Could you check a few things on this model? Use its own coordinates, in mm. A direction names the side the tool comes from. Round coordinates to 2 decimals unless told otherwise and drop trailing zeros. Loops run counter-clockwise (first coordinate to the right, second up) from the corner with the lowest first, then second, coordinate; pieces in that order, holes last. Notation, with made-up numbers: (22, 38) -> (74, 38) arc R21 cw to (74, 55) -> close; hole circle Ø5 at (21.5, -34). An arc over 180 degrees is marked (long way). One line per item, written item: value.
from build123d import *

# Parameters (mm, degrees)
BOSS_EXTRUDE1_DEPTH      = 17
SKETCH4_W                = 2.55
SKETCH4_H                = 15.3
SKETCH4_H_2              = 13.3
BOSS_EXTRUDE4_DEPTH      = 5
CHAMFER1_SIZE            = 0.6
SKETCH2_W                = 27.1
SKETCH2_H                = 15.3
BOSS_EXTRUDE2_DEPTH      = 2
SKETCH3_R                = 2.4
BOSS_EXTRUDE3_DEPTH      = 6
SKETCH5_R                = 0.75
CUT_EXTRUDE1_DEPTH       = 6
CUT_EXTRUDE2_REACH       = 41.661
SKETCH7_W                = 10
SKETCH7_H                = 2
BOSS_EXTRUDE5_DEPTH      = 45
BOSS_EXTRUDE5_DEPTH_BACK = 45
BOSS_EXTRUDE6_START      = -2
BOSS_EXTRUDE6_DEPTH      = 2
CHAMFER2_SIZE            = 0.6
CHAMFER4_SIZE            = 1
CHAMFER5_SIZE            = 0.8
BOSS_EXTRUDE7_START      = -3
BOSS_EXTRUDE7_DEPTH      = 3.6
LPATTERN1_COUNT          = 7
LPATTERN1_PITCH          = 14.6
FILLET1_R                = 5


with BuildPart() as part:
    # Sketch1 → Boss-Extrude1 (new body)
    with BuildSketch(Plane(origin=(0, 0, 0), x_dir=(1, 0, 0), z_dir=(0, 1, 0))):
        Polygon((-6.3, 5.3), (-6.3, -7), (-8.3, -7), (-8.3, 8.3), (18.8, 8.3), (18.8, -7), (16.8, -7), (16.8, 5.3), align=None)
    extrude(amount=-BOSS_EXTRUDE1_DEPTH)

    # Sketch4 → Boss-Extrude4 (add)
    with BuildSketch(Plane(origin=(0, 0, 0), x_dir=(1, 0, 0), z_dir=(0, 1, 0))):
        with Locations((-9.575, 0.65)):
            Rectangle(SKETCH4_W, SKETCH4_H)
        with Locations((20.075, -0.35)):
            Rectangle(SKETCH4_W, SKETCH4_H_2)
    extrude(amount=-BOSS_EXTRUDE4_DEPTH)

    # Chamfer1
    chamfer1_edges = [part.edges().sort_by_distance(p)[0] for p in [
        (16.8, 0, 0.85),
        (5.25, 0, -5.3),
        (-6.3, 0, 0.85),
    ]]
    chamfer(chamfer1_edges, length=CHAMFER1_SIZE)

    # Sketch2 → Boss-Extrude2 (add)
    with BuildSketch(Plane.XZ.offset(17)):
        with Locations((5.25, -0.65)):
            Rectangle(SKETCH2_W, SKETCH2_H)
    extrude(amount=BOSS_EXTRUDE2_DEPTH)

    # Sketch3 → Boss-Extrude3 (add)
    with BuildSketch(Plane.XZ.offset(19)):
        with Locations(Location((0, 1, 0), (0, 0, 270))):
            Circle(SKETCH3_R)
    extrude(amount=BOSS_EXTRUDE3_DEPTH)

    # Sketch5 → Cut-Extrude1 (cut)
    with BuildSketch(Plane(origin=(0, 0, 0), x_dir=(1, 0, 0), z_dir=(0, 1, 0))):
        with Locations(Location((-8.55, -1, 0), (0, 0, 270))):
            Circle(SKETCH5_R)
        with Locations(Location((19.05, -1, 0), (0, 0, 270))):
            Circle(SKETCH5_R)
    extrude(amount=-CUT_EXTRUDE1_DEPTH, mode=Mode.SUBTRACT)

    # Sketch7 → Cut-Extrude2 (cut, up to next)
    with BuildSketch(Plane.ZY.offset(8.3), mode=Mode.PRIVATE) as cut_extrude2_sk1:
        with Locations((2, -11)):
            Rectangle(SKETCH7_W, SKETCH7_H)
    cut_extrude2_tool1 = extrude(cut_extrude2_sk1.sketch, amount=-CUT_EXTRUDE2_REACH, mode=Mode.PRIVATE) & part.part
    add(cut_extrude2_tool1.solids().sort_by_distance((-8.3, -11, 2))[0], mode=Mode.SUBTRACT)

    # Sketch8 → Boss-Extrude5 (add, two sides: drawn at the far end of the back side and taken through both)
    with BuildSketch(Plane(origin=(0, -4, 1), x_dir=(1, 0, 0), z_dir=(0, 1, 0)).offset(-BOSS_EXTRUDE5_DEPTH_BACK)):
        with BuildLine():
            Line((21.35, 9.3), (-4.65, 9.3))
            ThreePointArc((-4.65, 9.3), (-15.891202985, 16.685930347), (-13.574121194, 29.935373491))
            Line((-13.574121194, 29.935373491), (1.493248773, 45.965793394))
            Line((1.493248773, 45.965793394), (2.819234682, 48.836640198))
            Line((2.819234682, 48.836640198), (2.090579232, 49.521520651))
            Line((2.090579232, 49.521520651), (-15.031432094, 31.305134397))
            ThreePointArc((-15.031432094, 31.305134397), (-17.726893838, 15.892054353), (-4.65, 7.3))
            Line((-4.65, 7.3), (21.35, 7.3))
            Line((21.35, 7.3), (21.35, 9.3))
        make_face()
    extrude(amount=BOSS_EXTRUDE5_DEPTH + BOSS_EXTRUDE5_DEPTH_BACK)

    # Sketch11 → Boss-Extrude6 (add)
    with BuildSketch(Plane(origin=(0, 41, 0), x_dir=(1, 0, 0), z_dir=(0, 1, 0)).offset(BOSS_EXTRUDE6_START)):
        with BuildLine():
            Line((0.537054569, 46.868700502), (-15.031432094, 30.305134397))
            ThreePointArc((-15.031432094, 30.305134397), (-17.726893838, 14.892054353), (-4.65, 6.3))
            Line((-4.65, 6.3), (13.753385306, 6.3))
            ThreePointArc((13.753385306, 6.3), (4.636095939, 25.766936525), (0.537054569, 46.868700502))
        make_face()
    boss_extrude6 = extrude(amount=BOSS_EXTRUDE6_DEPTH)

    # Mirror1: Boss-Extrude6 across plane
    add(boss_extrude6.mirror(Plane(origin=(0, -4, 1), x_dir=(0, 0, 1), z_dir=(0, 1, 0))))

    # Chamfer2
    chamfer2_edges = [part.edges().sort_by_distance(p)[0] for p in [
        (0, -25, 3.4),
    ]]
    chamfer(chamfer2_edges, length=CHAMFER2_SIZE)

    # Chamfer4
    chamfer4_edges = [part.edges().sort_by_distance(p)[0] for p in [
        (21.35, -4, -8.3),
    ]]
    chamfer(chamfer4_edges, length=CHAMFER4_SIZE)

    # Chamfer5
    chamfer5_edges = [part.edges().sort_by_distance(p)[0] for p in [
        (8.35, -49, -6.3),
        (-17.726893838, -49, -14.892054353),
        (-6.470426431, -49, -39.413327524),
        (-6.470426431, 41, -39.413327524),
        (-17.726893838, 41, -14.892054353),
        (8.35, 41, -6.3),
    ]]
    chamfer(chamfer5_edges, length=CHAMFER5_SIZE)

    # Sketch12 → Boss-Extrude7 (add)
    with BuildSketch(Plane(origin=(0, 41, 0), x_dir=(1, 0, 0), z_dir=(0, 1, 0)).offset(BOSS_EXTRUDE7_START)):
        Polygon((-2.018703486, 44.14958795), (4.145220591, 50.707487001), (4.873876041, 50.022606548), (2.906784676, 45.009568392), (0.167262864, 42.094946591), align=None)
    boss_extrude7 = extrude(amount=BOSS_EXTRUDE7_DEPTH)

    # LPattern1: Boss-Extrude7 ×7
    with Locations(*[(0, -i * LPATTERN1_PITCH, 0) for i in range(1, LPATTERN1_COUNT)]):
        add(boss_extrude7)

    # Fillet1
    fillet1_edges = [part.edges().sort_by_distance(p)[0] for p in [
        (21.35, 41, -7.2),
        (21.35, -49, -7.2),
    ]]
    fillet(fillet1_edges, radius=FILLET1_R)


solid = part.part
(1) If we section it at A-A, the plane y = 33: Please give me the cut outline in (x, z), then the cut area to 3 significant figures.
Recorded:
outline: (-15.03, -30.31) -> (2.09, -48.52) -> (2.82, -47.84) -> (1.49, -44.97) -> (-13.57, -28.94) arc R12.25 cw to (-4.65, -8.3) -> (20.35, -8.3) -> (21.35, -7.3) -> (21.35, -6.3) -> (-4.65, -6.3) arc R14.25 ccw to start
area: 162 mm²
(2) For faces 5 (the face through (4.98, 39.99, -24.73)), 6 (the face through (3, -35, -46)), 7 (the face through (19.85, 39.57, -7.31)), which set-ups out of +Z, -Z, +X, -X, +Y, -Y let a thin tool reach every point of the face, with its end or its side?
Recorded:
face 5: +X, +Y, -Y
face 6: +X
face 7: +Z, -Z, +X, +Y
(3) Thinking about a two-plate mould opening in Z: for faces 1 (the face through (8, 20, -6.3)), 2 (the face through (-10.85, -2, 0)), 3 (the face through (3, 27, -46)), 4 (the face through (3, -31.4, -46)), which applies, released by +Z, released by -Z, zero draft, split by the parting line, or undercut?
Recorded:
face 1: released by +Z
face 2: zero draft
face 3: undercut
face 4: undercut
(4) I'm going to push flat-ended pins straight in: pin 1 Ø3.5 at (x, z) = (5.5, 3) entering from +Y; pin 2 Ø1 at (x, y) = (-7, -35.5) entering from -Z; pin 3 Ø1.3 at (x, z) = (19.5, -0.5) entering from -Y. Where does each tip first touch, or does it pass through?
Recorded:
pin 1: y = -17
pin 2: z = -39.38
pin 3: y = -5
(5) If we section it at B-B, the plane x = 15: Please give me the cut outline in (y, z).
Recorded:
outline: (-49, -8.3) -> (41, -8.3) -> (41, -7.1) -> (40.2, -6.3) -> (0, -6.3) -> (0, -5.9) -> (-0.6, -5.3) -> (-17, -5.3) -> (-17, 7) -> (-19, 7) -> (-19, -6.3) -> (-48.2, -6.3) -> (-49, -7.1) -> close
(6) If I drill on L1, parallel to X at y = -1.75, z = 1; L2, parallel to Z at x = 19.05, y = -1.55; L3, parallel to Z at x = -8.55, y = -2.75, over which ranges is the centre line in solid material (lowest first)?
Recorded:
L1: -10.85 to -9.3, -7.8 to -6.3, 16.8 to 18.3, 19.8 to 21.35
L2: -8.3 to 0.25, 1.75 to 7
L3: -37.2 to -34.28, -8.94 to 0.25, 1.75 to 7
(7) If we section it at C-C, the plane z = -39: Please give me the cut outline in (x, y), then the cut area to 3 significant figures.
Recorded:
outline: (-6.86, -48.2) -> (-5.76, -49) -> (1.44, -49) -> (1.44, -47) -> (-4.11, -47) -> (-4.11, 39) -> (1.44, 39) -> (1.44, 41) -> (-5.76, 41) -> (-6.86, 40.2) -> close
area: 268 mm²
(8) If we section it at D-D, the plane x = 7: Please give me the cut outline in (y, z), then the cut area to 3 significant figures.
Recorded:
outline: (-49, -19.37) -> (-47, -19.37) -> (-47, -8.3) -> (39, -8.3) -> (39, -19.37) -> (41, -19.37) -> (41, -7.1) -> (40.2, -6.3) -> (0, -6.3) -> (0, -5.9) -> (-0.6, -5.3) -> (-17, -5.3) -> (-17, 7) -> (-19, 7) -> (-19, -6.3) -> (-48.2, -6.3) -> (-49, -7.1) -> close
area: 267 mm²
